For this review, take the finished solid that the model builds, in its own axes (mm). A direction names the side the tool comes from. Coordinates: 2 decimals unless noted, no trailing zeros. Write each loop counter-clockwise with the first axis right and the second up, starting at its lowest first coordinate (ties: lowest second). Pieces come first, ordered by that corner, then holes. Notation, with made-up numbers: M 28,6 L 43,6 A29 ccw 43,28 Z; hole C -8.5,70 d9. An arc over 180 degrees is marked long. One line per question, with ' | ' between items.
from build123d import *

# Parameters (mm, degrees)
F0_W     = 3
F0_H     = 20
F1_DEPTH = 3
F3_DEPTH = 3
F4_START = -17
F4_DEPTH = 3


with BuildPart() as f1:
    # F0 (on Top) → F1 (new body)
    with BuildSketch(Plane.XY):
        with Locations((1.5, 10)):
            Rectangle(F0_W, F0_H)
    extrude(amount=F1_DEPTH)



with BuildPart() as f1b:
    # F0 (on Top) → F1, piece 2 (new body)
    with BuildSketch(Plane.XY):
        with Locations((19.4732441902, 10)):
            Rectangle(F0_W, F0_H)
    extrude(amount=F1_DEPTH)


with BuildPart() as f1_1:
    add(f1.part)

    add(f1b.part)  # F3 merges F1b
    # F2 (on Front) → F3 (join)
    with BuildSketch(Plane.XZ):
        with BuildLine():
            ThreePointArc((2.9794946313, 2.1942069288), (10.4704971824, 3.8575045035), (17.9987903684, 2.37208209))
            Line((17.9987903684, 2.37208209), (18.889406696, 2.9833931476))
            ThreePointArc((18.889406696, 2.9833931476), (10.4870498812, 4.9495737182), (2.087746514, 2.970389789))
            Line((2.087746514, 2.970389789), (2.9794946313, 2.1942069288))
        make_face()
    extrude(amount=-F3_DEPTH)

    # F2 (on Front) → F4 (join)
    with BuildSketch(Plane.XZ.offset(F4_START)):
        with BuildLine():
            ThreePointArc((2.9794946313, 2.1942069288), (10.4704971824, 3.8575045035), (17.9987903684, 2.37208209))
            Line((17.9987903684, 2.37208209), (18.889406696, 2.9833931476))
            ThreePointArc((18.889406696, 2.9833931476), (10.4870498812, 4.9495737182), (2.087746514, 2.970389789))
            Line((2.087746514, 2.970389789), (2.9794946313, 2.1942069288))
        make_face()
    extrude(amount=-F4_DEPTH)


solid = f1_1.part
1) We need section D-D on x = 18.25. State the section outline as (y, z) points, then the cut area to 3 significant figures.
Responses:
outline: M 0,0 L 20,0 L 20,3.29 L 17,3.29 L 17,3 L 3,3 L 3,3.29 L 0,3.29 Z | area: 61.7 mm^2
2) Insertion check: pin 1 Ø12 at (x, y) = (18.5, 15.5) entering from +Z; pin 2 Ø3.5 at (x, y) = (1, 13) entering from +Z. Each pin has a flat end and moves straight along its axis. Give the tip position at first contact, or say it passes through.
Responses:
pin 1: z = 4.82 | pin 2: z = 3
3) The part is to be moulded in two halves that separate along X. For faces 6 (the flat face through (17.973, 10, 1)), 7 (the cylindrical face through (10.62, 1.48, 4.95)), 8 (the flat face through (1, 10, 0)), say which applies: +X half, -X half, draft (parallel to the pull), parting line (faces both ways), or undercut.
Responses:
face 6: undercut | face 7: parting line | face 8: draft
4) Machinability: for faces 1 (the flat face through (10, 0, 4)), 2 (the flat face through (1, 10, 3)), 3 (the flat face through (19, 10, 3)), 4 (the flat face through (3, 10, 1)), 5 (the cylindrical face through (10.36, 1.479, 3.856)), which of the approach directions +Z, -Z, +X, -X, +Y, -Y give a long, thin tool a straight path to every point of the face, cutting with its end or side? Answer none if there is none.
Responses:
face 1: +Z, -Z, +X, -X, -Y | face 2: +Z, -X | face 3: +Z, +X | face 4: -Z | face 5: -Z, +Y, -Y
5) We need section C-C on z = 3.6. State the section outline as (x, y) points, then the cut area to 3 significant figures.
Responses:
outline: M 3.49,0 L 7.59,0 L 7.59,3 L 3.49,3 Z; M 3.49,17 L 7.59,17 L 7.59,20 L 3.49,20 Z; M 13.79,0 L 17.51,0 L 17.51,3 L 13.79,3 Z; M 13.79,17 L 17.51,17 L 17.51,20 L 13.79,20 Z | area: 46.9 mm^2
6) We need section B-B on x = 6.75. State the section outline as (y, z) points.
Responses:
outline: M 0,3.44 L 3,3.44 L 3,4.57 L 0,4.57 Z; M 17,3.44 L 20,3.44 L 20,4.57 L 17,4.57 Z
7) To check wall thickness, follow line 1 along X through (y, z) = (10.75, 1); line 2 along Z through (x, y) = (1.25, 2.5); line 3 along Y through (x, z) = (15.5, 3.6). State the ranges of each line that lie inside material, in increasing order. Write a range as [from, to].
Responses:
line 1: [0, 3], [17.97, 20.97] | line 2: [0, 3] | line 3: [0, 3], [17, 20]
8) We need section A-A on y = 15. State the section outline as (x, z) points, then the cut area to 3 significant figures.
Responses:
outline: M 0,0 L 3,0 L 3,3 L 0,3 Z; M 17.97,0 L 20.97,0 L 20.97,3 L 17.97,3 Z | area: 18.0 mm^2
